Autodesk Inventor part; units mm, degrees
ref_plane "YZ Plane" through (0, 0, 0) normal (1, 0, 0) x (0, 1, 0)
ref_plane "XZ Plane" through (0, 0, 0) normal (0, 1, 0) x (-1, 0, 0)
ref_plane "XY Plane" through (0, 0, 0) normal (0, 0, 1) x (1, 0, 0)
sketch "Szkic1" plane through (0, 0, 0) normal (0, 1, 0) x (-1, 0, 0)
  circle A0 centre (0, 0) radius 50
  circle A1 centre (0, 40) radius 3
  circle A2 centre (0, -40) radius 3
  circle A3 centre (40, 0) radius 3
  circle A4 centre (-40, 0) radius 3
  circle A5 centre (0, 0) radius 20
  dimension "d0" = 100
  dimension "d1" = 6
  dimension "d2" = 6
  dimension "d3" = 6
  dimension "d4" = 6
  dimension "d5" = 40
  dimension "d6" = 80
  dimension "d7" = 40
  dimension "d8" = 80
  dimension "d9" = 40
extrude "Wyciągnięcie proste1" add sketch "Szkic1" along normal blind 5
sketch "Szkic2" plane through (0, 5, 0) normal (0, 1, 0) x (1, 0, 0)
  point P0 (0, 0)
sketch "Szkic3" plane through (0, 5, 0) normal (0, 1, 0) x (1, 0, 0)
  circle A0 centre (0, 0) radius 20
  circle A1 centre (0, 0) radius 5
  dimension "d12" = 40
  dimension "d13" = 10
extrude "Wyciągnięcie proste2" add sketch "Szkic3" along normal blind 2.5 and the other way blind 5
thread "Gwint1"
thread "Gwint2"
thread "Gwint3"
thread "Gwint4"
thread "Gwint5"
properties part number "płytka"
The model under review builds one solid part; all positions refer to its coordinate system, in mm. A direction names the side the tool comes from. Round coordinates to 2 decimals unless told otherwise and drop trailing zeros. Write each loop counter-clockwise with the first axis right and the second up, starting at its lowest first coordinate (ties: lowest second). Pieces come first, ordered by that corner, then holes. Notation, with made-up numbers: (70.5, 22) -> (91.5, 22) arc R25 cw to (91.5, 52) -> close; hole circle Ø8 at (1, 47). An arc over 180 degrees is marked (long way). Answer as a JSON object with one key per item and string values.
1. We need section B-B on z = -40. State the section outline as (x, y) points, and give its area (3 significant figures).
Results found:
{"outline": "(-30, 0) -> (-3, 0) -> (-3, 5) -> (-30, 5) -> close; (3, 0) -> (30, 0) -> (30, 5) -> (3, 5) -> close", "area": "270 mm^2"}
2. The part is to be moulded in two halves that separate along X. For faces 1 (the face through (4, 7.5, 4)), 2 (the face through (0, 2, 37)), 3 (the face through (-37, 2, 0)), 4 (the face through (-47.69, 2.46, -15.02)), say which applies: pulls with the +X half, pulls with the -X half, needs draft (parallel to the pull), parting line crosses it, or undercut.
Results found:
{"face 1": "needs draft", "face 2": "undercut", "face 3": "undercut", "face 4": "parting line crosses it"}
3. We need section D-D on x = 40. State the section outline as (y, z) points.
Results found:
{"outline": "(0, -30) -> (5, -30) -> (5, -3) -> (0, -3) -> close; (0, 3) -> (5, 3) -> (5, 30) -> (0, 30) -> close"}
4. We need section A-A on z = 0. State the section outline as (x, y) points, and give its area (3 significant figures).
Results found:
{"outline": "(-50, 0) -> (-43, 0) -> (-43, 5) -> (-50, 5) -> close; (-37, 0) -> (-5, 0) -> (-5, 7.5) -> (-20, 7.5) -> (-20, 5) -> (-37, 5) -> close; (5, 0) -> (37, 0) -> (37, 5) -> (20, 5) -> (20, 7.5) -> (5, 7.5) -> close; (43, 0) -> (50, 0) -> (50, 5) -> (43, 5) -> close", "area": "465 mm^2"}
5. Machinability: for faces 5 (the face through (1, 5, -22)), 6 (the face through (0, 2, -43)), which of the approach directions +Z, -Z, +X, -X, +Y, -Y give a long, thin tool a straight path to every point of the face, cutting with its end or side? Answer none if there is none.
Results found:
{"face 5": "+Y", "face 6": "+Y, -Y"}
6. We need section C-C on x = 0. State the section outline as (y, z) points.
Results found:
{"outline": "(0, -50) -> (5, -50) -> (5, -43) -> (0, -43) -> close; (0, -37) -> (5, -37) -> (5, -20) -> (7.5, -20) -> (7.5, -5) -> (0, -5) -> close; (0, 5) -> (7.5, 5) -> (7.5, 20) -> (5, 20) -> (5, 37) -> (0, 37) -> close; (0, 43) -> (5, 43) -> (5, 50) -> (0, 50) -> close"}
7. To check wall thickness, follow line 1 along Z through (x, y) = (0, 2.6); line 2 along Y through (x, z) = (41, 5); line 3 along X through (y, z) = (5.5, 0). State the ranges of each line that lie inside material, in increasing order.
Results found:
{"line 1": "z = -50 to -43, -37 to -5, 5 to 37, 43 to 50", "line 2": "y = 0 to 5", "line 3": "x = -20 to -5, 5 to 20"}
8. Clearance check with flat-ended pins moving along their axes: pin 1 (8 mm diameter, centred on x = 0, z = -40, fed in from +Y); pin 2 (3.5 mm diameter, centred on x = 0, z = 40, fed in from +Y); pin 3 (2 mm diameter, centred on y = 1.5, z = 8.5, fed in from -X); pin 4 (4 mm diameter, centred on x = 5, y = 2, fed in from +Z). State where each tip first meets the part, or that it passes through.
Results found:
{"pin 1": "stops at y = 5", "pin 2": "passes through", "pin 3": "stops at x = -49.43", "pin 4": "stops at z = 49.91"}
